Source: CAD feature listing. Evaluate the final solid. Frame: model axes, mm. A direction names the side the tool comes from. Give positions to 0.01 mm unless a question says otherwise; leave off trailing zeros. Loops run counter-clockwise (first coordinate to the right, second up) from the corner with the lowest first, then second, coordinate; pieces in that order, holes last.
Autodesk Inventor part; units mm, degrees
ref_plane "Plan de courroie" through (0, 20.5, 11) normal (0, 0, 1) x (1, 0, 0)
ref_plane "YZ Plane" through (0, 0, 0) normal (1, 0, 0) x (0, 1, 0)
ref_plane "XZ Plane" through (0, 0, 0) normal (0, 1, 0) x (-1, 0, 0)
sketch "Esquisse principale" plane through (0, 0, 0) normal (1, 0, 0) x (0, 1, 0)
  line L0 (0, 22) -> (31.5, 22)
  line L1 (31.5, 22) -> (31.5, 15.8615)
  line L2 (31.5, 15.8615) -> (20.5, 12.4984)
  line L3 (20.5, 12.4984) -> (20.5, 9.5016)
  line L4 (20.5, 9.5016) -> (31.5, 6.1385)
  line L5 (31.5, 6.1385) -> (31.5, 0)
  line L6 (31.5, 0) -> (0, 0)
  line L7 (29.5, 15.25) -> (29.5, 6.75) construction
  line L8 (20.5, 11) -> (29.5, 11) construction
  line L9 (31.5, 15.8615) -> (31.5, 6.1385)
  line L10 (0, -3.2) -> (0, 19.2)
  line L11 (0, 0) -> (0, 22)
  dimension "d0" = 8.5
  dimension "d1" = 34
  dimension "d2" = 2
  dimension "d6" = 22
  dimension "d21" = 59
  dimension "d25" = 11
  dimension "d27" = 11
ref_plane "Plan de courroie" through (0, 20.5, 11) normal (0, 0, 1) x (1, 0, 0)
revolve "Corps" add sketch "Esquisse principale" angle 360 about axis through (0, 0, -10) along (0, 0, 1)
revolve "Bord" cut sketch "Esquisse principale" angle 360 about axis through (0, 0, -10) along (0, 0, 1) contours L9 L4 L3 L2
fillet "Congé externe" [suppressed]
fillet "Congé interne" [suppressed]
pattern_of_one "Réseau de bords"
sketch "Esquisse2" plane through (0, 0, 22) normal (0, 0, 1) x (1, 0, 0)
  circle A0 centre (0, 0) radius 31.5
hole "Perçage1" at (0, 0, 22) direction (0, 0, -1) diameter 35 depth 22
equation "\"d0\" = da_Bw"
equation "\"d1\" = da_Alfa"
equation "\"d2\" = da_c"
equation "\"d21\" = da_Dw"
equation "\"d25\" = da_Hd"
equation "\"d27\" = da_Se"
equation "\"da_r1\" = 0"
equation "\"da_r2\" = 0"
equation "\"d18\" = da_Sg"
equation "\"d5\" = da_Se"
equation "\"da_Bw\" = 8.5"
equation "\"da_Alfa\" = 34deg"
equation "\"da_c\" = 2"
equation "\"da_Dw\" = 59"
equation "\"da_Hd\" = 11"
equation "\"da_Se\" = 11"
equation "\"da_Sg\" = 12"
properties part number "Poulie à gorge2" material "Steel"
1) Cut plane C-C (z = 7). Return loops of the section in (x, y).
Checks:
outline: circle Ø57.36 at (0, 0); hole circle Ø35 at (0, 0)
2) Ray query, probe 1 along X at (y, z) = (0, 4.5); probe 2 along Z at (x, y) = (-25.5, 15); probe 3 along X at (y, z) = (3, 10.75). Return the intervals inside material, ascending.
Checks:
probe 1: x = -31.5 to -17.5, 17.5 to 31.5
probe 2: z = 0 to 6.72, 15.28 to 22
probe 3: x = -20.28 to -17.24, 17.24 to 20.28
3) Contact query for flat-ended pins moving along their axis: P1, Ø10, axis at x = 18, z = 10, coming from the +Y side; P2, Ø3, axis at y = 0, z = 18.5, coming from the -X side; P3, Ø2, axis at y = -8, z = 5, coming from the -X side. Output: stop coordinate, or through.
Checks:
P1: stops at y = 27.79
P2: stops at x = -31.5
P3: stops at x = -30.71
4) Pull-direction query (Z, two-part tool) for faces 3 (the flat face through (14, 14, 0)), 4 (the cylindrical face through (31.232, -4.101, 3.026)), 5 (the conical face through (-0.93, -21.17, 12.71)); classes: released by +Z, released by -Z, zero draft, split by the parting line, or undercut.
Checks:
face 3: released by -Z
face 4: zero draft
face 5: undercut
5) Cut plane A-A (x = 0). Return loops of the section in (y, z), and give its area (3 significant figures).
Checks:
outline: (-31.5, 0) - (-17.5, 0) - (-17.5, 22) - (-31.5, 22) - (-31.5, 15.86) - (-20.5, 12.5) - (-20.5, 9.5) - (-31.5, 6.14) - close; (17.5, 0) - (31.5, 0) - (31.5, 6.14) - (20.5, 9.5) - (20.5, 12.5) - (31.5, 15.86) - (31.5, 22) - (17.5, 22) - close
area: 476 mm2
6) Reachability of faces 1 (the cylindrical face through (10.648, 13.887, 10.846)), 2 (the conical face through (-20.684, -4.593, 9.291)) from +Z, -Z, +X, -X, +Y, -Y: full face, straight path, thin tool, end or side. Return the list, or none.
Checks:
face 1: +Z, -Z
face 2: none
